The model under review builds one solid part; all positions refer to its coordinate system, in mm. A direction names the side the tool comes from. Coordinates: 2 decimals unless noted, no trailing zeros. Loops run counter-clockwise (first coordinate to the right, second up) from the corner with the lowest first, then second, coordinate; pieces in that order, holes last. Notation, with made-up numbers: (-29.75, 29) - (-18.75, 29) arc R16 ccw to (-18.75, 58) - close; hole circle Ø10 at (56, 40). An arc over 180 degrees is marked (long way). Answer in a Markdown table with one row per item. Add a question column.
(1) We need section C-C on x = 233. Write out the cut boundary in (y, z), plus the area to 3 significant figures.
(2) For line 1 along X through (y, z) = (14.5, 4.5); line 2 along X through (y, z) = (11.65, 16.25); line 3 along Z through (x, y) = (275, 14), list the stretches that pass through material, from the lowest coordinate up.
(3) Mouldability with a two-part tool opening along Z and no side actions: class faces 6 (the flat face through (25, 5, 22.5)), 7 (the cylindrical face through (299.994, 24.65, 0.55)), 8 (the flat face through (176, 0, 0)) as +Z half, -Z half, draft (parallel to the pull), parting line (faces both ways), or undercut.
(4) Machinability: for faces 1 (the cylindrical face through (-13.887, 145.944, 10.648)), 2 (the flat face through (278, 40, -15)), 3 (the flat face through (136, 25, 25)), 4 (the flat face through (20, 27, 11)), 5 (the flat face through (27, 10, -12)), which of the approach directions +Z, -Z, +X, -X, +Y, -Y give a long, thin tool a straight path to every point of the face, cutting with its end or side? Answer none if there is none.
(5) For P1, Ø1.5, axis at y = 13, z = 7, coming from the +X side; P2, Ø10, axis at x = 252, z = 1, coming from the +Y side; P3, Ø24, axis at x = 275, z = 0, coming from the +Y side; P4, Ø2, axis at y = 123, z = -14, coming from the +X side, all flat-tipped, find the tip position at first contact; note any pin that passes through.
(6) We need section B-B on x = 4. Write out the cut boundary in (y, z), plus the area to 3 significant figures.
(7) We need section D-D on y = 90. Write out the cut boundary in (x, z).
(8) We need section A-A on y = 31.5. Write out the cut boundary in (x, z).
from build123d import *

# Parameters (mm, degrees)
RECTWITHARC_W              = 275
RECTWITHARC_H              = 50
ARMBASE_DEPTH              = 50
ARMCOLLAR_START            = 50
SKETCH5_R                  = 25
ARMCOLLAR_DEPTH            = 100
CUT_EXTRUDE1_REACH         = 152
SHAFTKEY_R                 = 17.5
HOLLOWMIDDLE_DEPTH         = 15
HOLLOWMIDDLE_DEPTH_BACK    = 26
J2SHAFTHOLE_R              = 15
JOINT2SHAFTHOLE_DEPTH      = 151
JOINT2SHAFTHOLE_DEPTH_BACK = 10
J2SHAFTCOUNTERSINK_START   = 50
SKETCH4_R                  = 20
J2SHAFTCOUNTERSINK_DEPTH   = 10
SKETCH6_R                  = 21
INNERDIAMETER_DEPTH        = 142
CUT_EXTRUDE11_DEPTH        = 10
CUT_EXTRUDE12_START        = 10
SKETCH9_W                  = 50
SKETCH9_H                  = 20
CUT_EXTRUDE12_DEPTH        = 5
CUT_EXTRUDE13_START        = 10
SKETCH11_R                 = 2.5
CUT_EXTRUDE13_DEPTH        = 5


with BuildPart() as part:
    # RectwithArc → ArmBase (new body)
    with BuildSketch(Plane(origin=(0, 0, 0), x_dir=(1, 0, 0), z_dir=(0, 1, 0))):
        with BuildLine():
            ThreePointArc((0, -25), (-25, 0), (0, 25))
            Line((0, 25), (0, -25))
        make_face()
        with Locations((137.5, 0)):
            Rectangle(RECTWITHARC_W, RECTWITHARC_H)
        with BuildLine():
            Line((275, 25), (275, -25))
            ThreePointArc((275, -25), (300, 0), (275, 25))
        make_face()
    extrude(amount=ARMBASE_DEPTH)

    # Sketch5 → ArmCollar (add)
    with BuildSketch(Plane(origin=(0, 0, 0), x_dir=(1, 0, 0), z_dir=(0, 1, 0)).offset(ARMCOLLAR_START)):
        Circle(SKETCH5_R)
    extrude(amount=ARMCOLLAR_DEPTH)

    # ShaftKey → Cut-Extrude1 (cut, up to next)
    with BuildSketch(Plane(origin=(0, 0, 0), x_dir=(1, 0, 0), z_dir=(0, 1, 0)), mode=Mode.PRIVATE) as cut_extrude1_sk1:
        Circle(SHAFTKEY_R)
    cut_extrude1_tool1 = extrude(cut_extrude1_sk1.sketch, amount=CUT_EXTRUDE1_REACH, mode=Mode.PRIVATE) & part.part
    add(cut_extrude1_tool1.solids().sort_by_distance((0, 0, 0))[0], mode=Mode.SUBTRACT)

    # Sketch1 → HollowMIddle (cut, two sides)
    with BuildSketch(Plane.XY) as hollowmiddle_sk:
        Polygon((20, 40), (250, 40), (250, 10), (70, 10), (70, 15), (20, 15), align=None)
    extrude(amount=HOLLOWMIDDLE_DEPTH, mode=Mode.SUBTRACT)
    extrude(hollowmiddle_sk.sketch, amount=-HOLLOWMIDDLE_DEPTH_BACK, mode=Mode.SUBTRACT)

    # J2ShaftHole → Joint2ShaftHole (cut, two sides)
    with BuildSketch(Plane(origin=(0, 0, 0), x_dir=(1, 0, 0), z_dir=(0, 1, 0))) as joint2shafthole_sk:
        with Locations((275, 0)):
            Circle(J2SHAFTHOLE_R)
    extrude(amount=JOINT2SHAFTHOLE_DEPTH, mode=Mode.SUBTRACT)
    extrude(joint2shafthole_sk.sketch, amount=-JOINT2SHAFTHOLE_DEPTH_BACK, mode=Mode.SUBTRACT)

    # Sketch4 → J2ShaftCounterSink (cut)
    with BuildSketch(Plane(origin=(0, 0, 0), x_dir=(1, 0, 0), z_dir=(0, 1, 0)).offset(J2SHAFTCOUNTERSINK_START)):
        with Locations((275, 0)):
            Circle(SKETCH4_R)
    extrude(amount=-J2SHAFTCOUNTERSINK_DEPTH, mode=Mode.SUBTRACT)

    # Sketch6 → InnerDiameter (cut)
    with BuildSketch(Plane(origin=(0, 0, 0), x_dir=(1, 0, 0), z_dir=(0, 1, 0))):
        Circle(SKETCH6_R)
    extrude(amount=INNERDIAMETER_DEPTH, mode=Mode.SUBTRACT)

    # Sketch10 → Cut-Extrude11 (cut)
    with BuildSketch(Plane(origin=(0, 0, 0), x_dir=(1, 0, 0), z_dir=(0, 1, 0))):
        with BuildLine():
            Line((0, 22.5), (50, 22.5))
            Line((50, 22.5), (50, -22.5))
            Line((50, -22.5), (0, -22.5))
            ThreePointArc((0, -22.5), (-22.5, 0), (0, 22.5))
        make_face()
    extrude(amount=CUT_EXTRUDE11_DEPTH, mode=Mode.SUBTRACT)

    # Sketch9 → Cut-Extrude12 (cut)
    with BuildSketch(Plane(origin=(0, 0, 0), x_dir=(1, 0, 0), z_dir=(0, 1, 0)).offset(CUT_EXTRUDE12_START)):
        with Locations((25, 0)):
            Rectangle(SKETCH9_W, SKETCH9_H)
    extrude(amount=CUT_EXTRUDE12_DEPTH, mode=Mode.SUBTRACT)

    # Sketch11 → Cut-Extrude13 (cut)
    with BuildSketch(Plane(origin=(0, 0, 0), x_dir=(1, 0, 0), z_dir=(0, 1, 0)).offset(CUT_EXTRUDE13_START)):
        with Locations((30, 16.25)):
            Circle(SKETCH11_R)
        with Locations((30, -16.25)):
            Circle(SKETCH11_R)
    extrude(amount=CUT_EXTRUDE13_DEPTH, mode=Mode.SUBTRACT)


solid = part.part
Outcome:
| question | item | result |
|---|---|---|
| 1 | outline | (0, -25) - (10, -25) - (10, 15) - (40, 15) - (40, -25) - (50, -25) - (50, 25) - (0, 25) - close |
| 1 | area | 1,300 mm² |
| 2 | line 1 | -24.59 to -20.51, 50 to 70, 250 to 260.69, 289.31 to 299.59 |
| 2 | line 2 | -19 to -13.3, 13.3 to 27.5, 32.5 to 294 |
| 2 | line 3 | -25 to -15, 15 to 25 |
| 3 | face 6 | undercut |
| 3 | face 7 | parting line |
| 3 | face 8 | draft |
| 4 | face 1 | +Y, -Y |
| 4 | face 2 | +Y |
| 4 | face 3 | +Z, +X, -X, +Y, -Y |
| 4 | face 4 | -Z |
| 4 | face 5 | -Y |
| 5 | P1 | x = 299.21 |
| 5 | P2 | y = 50 |
| 5 | P3 | through |
| 5 | P4 | x = 21.35 |
| 6 | outline | (0, -25) - (50, -25) - (50, -24.68) - (150, -24.68) - (150, -17.04) - (142, -17.04) - (142, -20.62) - (10, -20.62) - (10, -22.5) - (0, -22.5) - close; (0, 22.5) - (10, 22.5) - (10, 20.62) - (142, 20.62) - (142, 17.04) - (150, 17.04) - (150, 24.68) - (50, 24.68) - (50, 25) - (0, 25) - close |
| 6 | area | 1,270 mm² |
| 7 | outline | circle Ø50 at (0, 0); hole circle Ø42 at (0, 0) |
| 8 | outline | (0, -25) - (20, -25) - (20, -6.4) arc R21 cw (long way) to (20, 6.4) - (20, 15) - (250, 15) - (250, -25) - (275, -25) arc R25 ccw to (275, 25) - (0, 25) arc R25 ccw to start; hole circle Ø30 at (275, 0) |
